```python
from build123d import *

# Parameters (mm, degrees)
F0_W     = 151.4763683081
F0_H     = 87.5145420432
F1_DEPTH = 46.228
F3_DEPTH = 102.87
F5_DEPTH = 30.48
F6_W     = 9.5930825919
F6_H     = 18.165897578
F6_W_2   = 95.0514208525
F7_DEPTH = 6.35
F8_R     = 4.5954023878
F9_DEPTH = 52.324


with BuildPart() as f1:
    # F0 (on Top) → F1 (new body)
    with BuildSketch(Plane.XY):
        Rectangle(F0_W, F0_H)
    extrude(amount=F1_DEPTH)

    # F2 (on face) → F3 (cut)
    with BuildSketch(Plane.XZ.offset(43.7572710216)):
        Polygon((75.738184154, 46.228), (19.3132366985, 46.228), (75.738184154, 0), align=None)
    extrude(amount=-F3_DEPTH, mode=Mode.SUBTRACT)

    # F4 (on face) → F5 (cut)
    with BuildSketch(Plane.XZ.offset(43.7572710216)):
        Polygon((75.738184154, 0), (35.9745252221, 32.5776896214), (35.9745252221, 0), align=None)
    extrude(amount=-F5_DEPTH, mode=Mode.SUBTRACT)

    # F6 (on face) → F7 (cut)
    with BuildSketch(Plane.XY.offset(46.228)):
        with Locations((24.1097779945, 0)):
            Rectangle(F6_W, F6_H)
        with Locations((-28.2124737278, 0)):
            Rectangle(F6_W_2, F6_H)
    extrude(amount=-F7_DEPTH, mode=Mode.SUBTRACT)

    # F8 (on face) → F9 (cut)
    with BuildSketch(Plane(origin=(30.4192109251, 0, 37.1290641622), x_dir=(0.7735396624, 0, -0.6337478921), z_dir=(0.6337478921, 0, 0.7735396624))):
        with Locations((20.0625781017, 0.542650738)):
            Circle(F8_R)
        with Locations((20.032882325, 29.4986355108)):
            Circle(F8_R)
        with Locations((46.194882325, 29.4986355108)):
            Circle(F8_R)
        with Locations((46.2245781017, 0.542650738)):
            Circle(F8_R)
    extrude(amount=-F9_DEPTH, mode=Mode.SUBTRACT)


solid = f1.part
```
Read the model definition and answer for the solid it produces. Units are mm, in the model's axes. A direction names the side the tool comes from. Give positions to 0.01 mm unless a question says otherwise; leave off trailing zeros. Write each loop counter-clockwise with the first axis right and the second up, starting at its lowest first coordinate (ties: lowest second). Pieces come first, ordered by that corner, then holes. Notation, with made-up numbers: (52, 75.25) -> (101, 75.25) arc R15 cw to (101, 95.25) -> close; hole circle Ø1 at (65, 13). An arc over 180 degrees is marked (long way). Answer in a Markdown table with one row per item.
1) Section B-B on y = -36 is taken. Give the vertices of the cut face in (x, z), plus the area to 3 significant figures.
Results list:
| item | result |
|---|---|
| outline | (-75.74, 0) -> (35.97, 0) -> (35.97, 32.58) -> (19.31, 46.23) -> (-75.74, 46.23) -> close |
| area | 5,050 mm^2 |
2) Determine the mould class of faces 1 (the flat face through (-29, 27, 46.228)), 2 (the flat face through (35.975, -29, 17)), 3 (the cylindrical face through (31.3, 0.74, 13.79)) for opening direction X: released by +X, released by -X, zero draft, split by the parting line, or undercut.
Results list:
| item | result |
|---|---|
| face 1 | zero draft |
| face 2 | released by +X |
| face 3 | undercut |
3) Straight lines are drawn through the part: line 1 (Z direction, x = 1, y = -7); line 2 (X direction, y = -19, z = 6); line 3 (X direction, y = 2, z = 18). For each, find the intervals that lie inside material, in ascending order. Write a range as [from, to].
Results list:
| item | result |
|---|---|
| line 1 | [0, 39.88] |
| line 2 | [-75.74, 35.97] |
| line 3 | [-75.74, 35.05], [46.32, 53.77] |
4) Each of these flat-tipped pins is pushed along its axis until it touches: pin 1 Ø16.5 at (x, z) = (57.5, 20) entering from -Y; pin 2 Ø5 at (y, z) = (-31.5, 11) entering from +X; pin 3 Ø9 at (x, y) = (-36, 4) entering from +Z. Where does it stop, or does it pass through?
Results list:
| item | result |
|---|---|
| pin 1 | y = -13.28 |
| pin 2 | x = 35.97 |
| pin 3 | z = 39.88 |
5) A tool of negligible diameter and unlimited length cuts with its end or side. For faces 4 (the flat face through (-25, 0, 39.878)), 5 (the flat face through (47, -13.277, 9)), 6 (the cylindrical face through (59.2, 29.7, 6.61)), from which of +Z, -Z, +X, -X, +Y, -Y can it reach the whole face along a straight path? Write none if from no direction.
Results list:
| item | result |
|---|---|
| face 4 | +Z, +X, -X |
| face 5 | +Z, -Z, +X, -Y |
| face 6 | none |
6) Section C-C on x = 63.5 is taken. Count the separate pieces of the cut face and the enclosed holes in it, plus the area to 3 significant figures.
Results list:
| item | result |
|---|---|
| separate pieces | 3 |
| enclosed holes | 0 |
| area | 404 mm^2 |
7) Section A-A on x = -44 is taken. Give the vertices of the cut face in (y, z), plus the area to 3 significant figures.
Results list:
| item | result |
|---|---|
| outline | (-43.76, 0) -> (43.76, 0) -> (43.76, 46.23) -> (9.08, 46.23) -> (9.08, 39.88) -> (-9.08, 39.88) -> (-9.08, 46.23) -> (-43.76, 46.23) -> close |
| area | 3,930 mm^2 |
